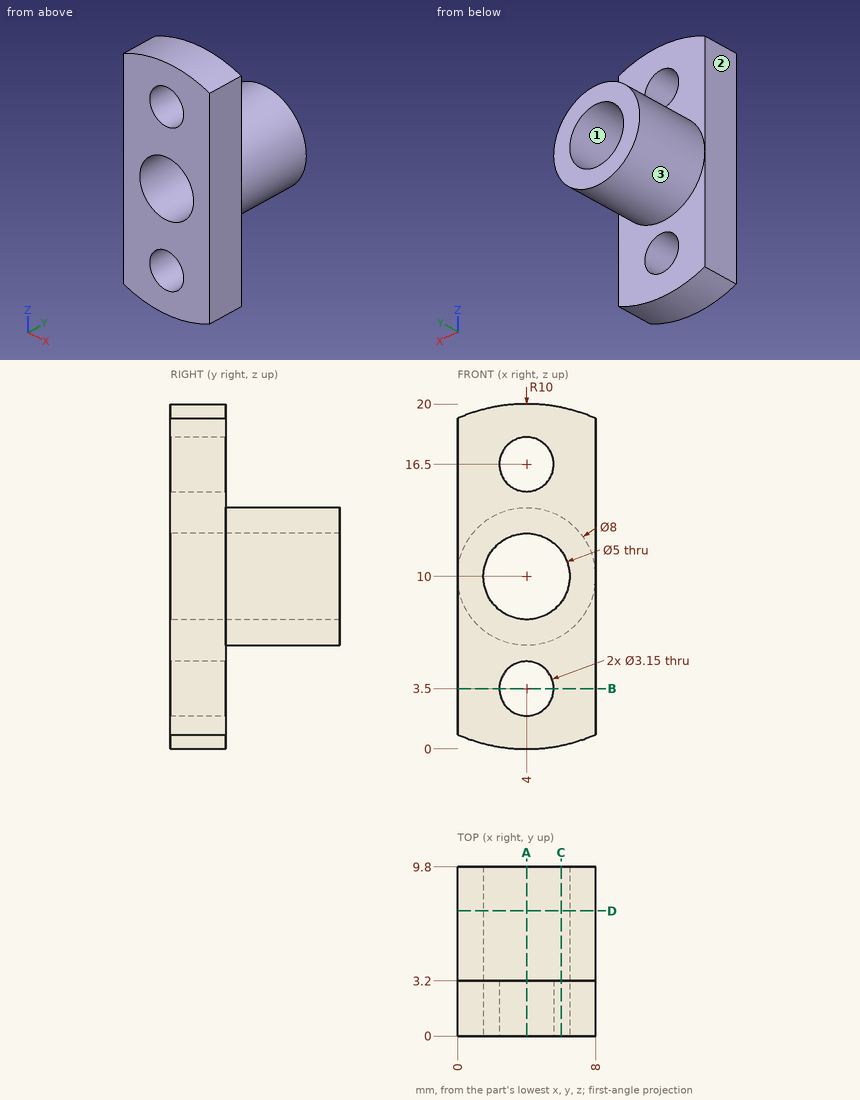
The drawing under review shows one solid part. Ordinate dimensions are in mm from its lowest x, y, z. Round coordinates to 2 decimals unless told otherwise and drop trailing zeros. Order: outer loops, then holes, each group sorted by start corner. A loop starts at its lowest first (then second) coordinate and runs counter-clockwise, first axis right, second up. Notation, with made-up numbers: (36, 42.25) -> (89, 42.25) arc R32 ccw to (89, 81.25) -> close; hole circle Ø7 at (-21, 19.25). An arc over 180 degrees is marked (long way). Use a Markdown table: item, result.
Item 1: Take a section at D-D (y = 7.25). State the section outline as (x, z) points.
Resolved:
| item | result |
|---|---|
| outline | circle Ø8 at (4, 10); hole circle Ø5 at (4, 10) |
Item 2: For pin 1 (3 mm diameter, centred on x = 4.5, y = 7, fed in from +Z); pin 2 (2 mm diameter, centred on x = 2, y = 3, fed in from +Z); pin 3 (3 mm diameter, centred on x = 5.5, y = 8, fed in from -Z), all flat-tipped, find the tip position at first contact; note any pin that passes through.
Resolved:
| item | result |
|---|---|
| pin 1 | stops at z = 14 |
| pin 2 | stops at z = 19.95 |
| pin 3 | stops at z = 6 |
Item 3: For line 1 along X through (y, z) = (2.4, 16.5) (3 decimals); line 2 along X through (y, z) = (3.5, 10); line 3 along Y through (x, z) = (6.5, 2.25), list the stretches that pass through material, from the lowest coordinate up. Write a range as [from, to].
Resolved:
| item | result |
|---|---|
| line 1 | x = [0, 2.425], [5.575, 8] |
| line 2 | x = [0, 1.5], [6.5, 8] |
| line 3 | y = [0, 3.2] |
Item 4: Take a section at A-A (x = 4). State the section outline as (y, z) points (3 decimals).
Resolved:
| item | result |
|---|---|
| outline | (0, 0) -> (3.2, 0) -> (3.2, 1.925) -> (0, 1.925) -> close; (0, 5.075) -> (3.2, 5.075) -> (3.2, 6) -> (9.8, 6) -> (9.8, 7.5) -> (0, 7.5) -> close; (0, 12.5) -> (9.8, 12.5) -> (9.8, 14) -> (3.2, 14) -> (3.2, 14.925) -> (0, 14.925) -> close; (0, 18.075) -> (3.2, 18.075) -> (3.2, 20) -> (0, 20) -> close |
Item 5: Take a section at B-B (z = 3.5). State the section outline as (x, y) points (3 decimals).
Resolved:
| item | result |
|---|---|
| outline | (0, 0) -> (2.425, 0) -> (2.425, 3.2) -> (0, 3.2) -> close; (5.575, 0) -> (8, 0) -> (8, 3.2) -> (5.575, 3.2) -> close |
Item 6: Draft analysis for pull direction X (two halves, no side actions). For the marked faces 1, 2 and 3, state which applies: +X half, -X half, draft (parallel to the pull), parting line (faces both ways), or undercut.
Resolved:
| item | result |
|---|---|
| face 1 | undercut |
| face 2 | -X half |
| face 3 | parting line |
Item 7: Take a section at C-C (x = 6). State the section outline as (y, z) points, plus the area to 3 significant figures.
Resolved:
| item | result |
|---|---|
| outline | (0, 0.2) -> (3.2, 0.2) -> (3.2, 6.54) -> (9.8, 6.54) -> (9.8, 8.5) -> (0, 8.5) -> close; (0, 11.5) -> (9.8, 11.5) -> (9.8, 13.46) -> (3.2, 13.46) -> (3.2, 19.8) -> (0, 19.8) -> close |
| area | 79.0 mm² |
